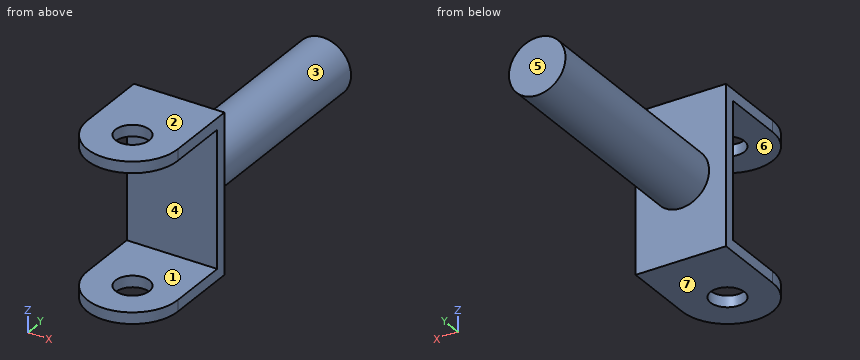
```python
from build123d import *

# Parameters (mm, degrees)
ESQUISSE1_R      = 1.5
EXTRUSION1_DEPTH = 14
ESQUISSE2_R      = 2.5
EXTRUSION2_DEPTH = 20
ESQUISSE5_W      = 12
ESQUISSE5_H      = 9.78359792
EXTRUSION4_DEPTH = 20


with BuildPart() as part:
    # Esquisse1 → Extrusion1 (new body)
    with BuildSketch(Plane.XY):
        with BuildLine():
            Line((0, 3.5), (0, 10))
            Line((0, 10), (8, 10))
            Line((8, 10), (8, 3.5))
            ThreePointArc((8, 3.5), (4, -0.5), (0, 3.5))
        make_face()
        with Locations((4, 3.5)):
            Circle(ESQUISSE1_R, mode=Mode.SUBTRACT)
    extrude(amount=EXTRUSION1_DEPTH)

    # Esquisse2 → Extrusion2 (add)
    with BuildSketch(Plane(origin=(0, 10, 0), x_dir=(1, 0, 0), z_dir=(0, 1, 0))):
        with Locations((4, -7)):
            Circle(ESQUISSE2_R)
    extrude(amount=EXTRUSION2_DEPTH)

    # Esquisse5 → Extrusion4 (cut)
    with BuildSketch(Plane.ZY):
        with Locations((7, 4.10820104)):
            Rectangle(ESQUISSE5_W, ESQUISSE5_H)
    extrude(amount=-EXTRUSION4_DEPTH, mode=Mode.SUBTRACT)


solid = part.part
```
Work out the finished part from the listing and answer in its coordinate system (mm). Face numbers are marked on the shaded views. A direction names the side the tool comes from. Give positions to 0.01 mm unless a question says otherwise; leave off trailing zeros. Loops run counter-clockwise (first coordinate to the right, second up) from the corner with the lowest first, then second, coordinate; pieces in that order, holes last. Notation, with made-up numbers: (27.5, 73.5) - (47.5, 73.5) arc R22 ccw to (47.5, 97.5) - close; hole circle Ø1 at (-6, 61). An arc over 180 degrees is marked (long way). One line per question, with ' | ' between items.
(1) The part is cut by section C-C (z = 7). Write down the section's boundary in (x, y), then the cut area to 3 significant figures.
Recorded:
outline: (0, 9) - (8, 9) - (8, 10) - (6.5, 10) - (6.5, 30) - (1.5, 30) - (1.5, 10) - (0, 10) - close | area: 108 mm²
(2) Straight lines are drawn through the part: probe 1 along X at (y, z) = (3.5, 13.65); probe 2 along Z at (x, y) = (0.5, 8.5); probe 3 along Y at (x, z) = (4, 0.45). For each, find the intervals that lie inside material, in ascending order.
Recorded:
probe 1: x = 0 to 2.5, 5.5 to 8 | probe 2: z = 0 to 1, 13 to 14 | probe 3: y = -0.5 to 2, 5 to 10
(3) The part is cut by section B-B (x = 4). Write down the section's boundary in (y, z), then the cut area to 3 significant figures.
Recorded:
outline: (-0.5, 0) - (2, 0) - (2, 1) - (-0.5, 1) - close; (-0.5, 13) - (2, 13) - (2, 14) - (-0.5, 14) - close; (5, 0) - (10, 0) - (10, 4.5) - (30, 4.5) - (30, 9.5) - (10, 9.5) - (10, 14) - (5, 14) - (5, 13) - (9, 13) - (9, 1) - (5, 1) - close | area: 127 mm²
(4) The part is cut by section A-A (y = 8). Write down the section's boundary in (x, z), then the cut area to 3 significant figures.
Recorded:
outline: (0, 0) - (8, 0) - (8, 1) - (0, 1) - close; (0, 13) - (8, 13) - (8, 14) - (0, 14) - close | area: 16.0 mm²
(5) The mould has two halves that part along Z. Classify the marked faces 4, 5, 6 and 7: +Z half, -Z half, draft (parallel to the pull), parting line (faces both ways), or undercut.
Recorded:
face 4: undercut | face 5: draft | face 6: undercut | face 7: -Z half
(6) Each of these flat-tipped pins is pushed along its axis until it touches: pin 1 Ø1 at (x, z) = (1.5, 2.5) entering from -Y; pin 2 Ø2 at (y, z) = (26.5, 9) entering from +X; pin 3 Ø6 at (y, z) = (16.5, 5) entering from -X. Where does it stop, or does it pass through?
Recorded:
pin 1: stops at y = 9 | pin 2: stops at x = 6.29 | pin 3: stops at x = 1.5
(7) A tool of negligible diameter and unlimited length cuts with its end or side. For the marked faces 1, 2 and 3, from which of +Z, -Z, +X, -X, +Y, -Y can it reach the whole face along a straight path? Write none if from no direction.
Recorded:
face 1: +X, -X, -Y | face 2: +Z, +X, -X, +Y, -Y | face 3: +Y
(8) The part is cut by section D-D (x = 7). Write down the section's boundary in (y, z).
Recorded:
outline: (0.85, 0) - (10, 0) - (10, 14) - (0.85, 14) - (0.85, 13) - (9, 13) - (9, 1) - (0.85, 1) - close
